Part model, mm, in its own coordinate system. A direction names the side the tool comes from. Round coordinates to 2 decimals unless told otherwise and drop trailing zeros. Order: outer loops, then holes, each group sorted by start corner. A loop starts at its lowest first (then second) coordinate and runs counter-clockwise, first axis right, second up. Notation, with made-up numbers: (49.5, 85) - (53.5, 85) arc R14 ccw to (53.5, 109) - close; hole circle Ø3 at (-6, -28.5). An arc over 180 degrees is marked (long way). Answer as a JSON object with one key per item and string values.
Autodesk Inventor part; units mm, degrees
ref_plane "Work Plane1" through (0, -10, 0) normal (0, 1, 0) x (-1, 0, 0)
ref_plane "YZ Plane" through (0, 0, 0) normal (1, 0, 0) x (0, 1, 0)
ref_plane "XY Plane" through (0, 0, 0) normal (0, 0, 1) x (1, 0, 0)
sketch "Sketch1" plane through (0, 0, 0) normal (1, 0, 0) x (0, 1, 0)
  circle A0 centre (0, 0) radius 7.5
  arc A1 (-3.1515, -19.7501) -> (-1.8071, 19.9182) centre (0, 0) ccw
  line L0 (-40, 20.115) -> (-40, -20.115)
  arc A2 (-40, 20.115) -> (-1.8071, 19.9182) centre (-19.8777, 219.1002) ccw
  arc A3 (-3.1515, -19.7501) -> (-40, -20.115) centre (-19.6039, -219.0723) ccw
  point P0 (-40, 0)
  dimension "d6" = 15
  dimension "d7" = 40
  dimension "d30" = 40.23
  dimension "d31" = 40
  dimension "d32" = 200
  dimension "d33" = 200
  dimension "d34" = 438.1724
  dimension "d35" = 219.0723
extrude "Extrusion1" add sketch "Sketch1" along normal mid plane 28
sketch "Sketch3" plane through (0, 0, 0) normal (0, 0, 1) x (1, 0, 0)
  line L0 (-14, 20) -> (14, 20) construction
  line L1 (-14, -3.1515) -> (14, -3.1515) construction
  line L2 (14, -40) -> (14, -3.1515) construction
  line L3 (14, -40) -> (-14, -40) construction
  line L4 (-14, -3.1515) -> (-14, -40) construction
  line L5 (-9, 20) -> (9, 20)
  line L6 (9, 20) -> (9, -10)
  line L7 (9, -10) -> (-9, -10)
  line L8 (-9, -10) -> (-9, 20)
  point P0 (0, 0)
  point P1 (0, 20)
  point P2 (0, 20)
  dimension "d19" = 18
  dimension "d21" = 10
extrude "Extrusion3" cut sketch "Sketch3" along normal through all both and the other way through all
ref_plane "Work Plane1" through (0, -10, 0) normal (0, 1, 0) x (-1, 0, 0)
sketch "Sketch5" plane through (0, -10, 0) normal (0, 1, 0) x (-1, 0, 0)
  circle A0 centre (0, 0) radius 2.75
  circle A1 centre (0, 0) radius 4.3
  dimension "d37" = 5.5
  dimension "d38" = 8.6
extrude "Extrusion6" cut sketch "Sketch5" against normal blind 3.2 contours A0 | A1
extrude "Extrusion7" cut sketch "Sketch5" against normal through all contours A0
properties part number "cabeza_obj1"
Item 1: Cut at A-A (z = 0). Write the cut outline in (x, y).
Taken from the geometry:
{"outline": "(-14, -40) - (-2.75, -40) - (-2.75, -13.2) - (-4.3, -13.2) - (-4.3, -10) - (-9, -10) - (-9, -7.5) - (-14, -7.5) - close; (-14, 7.5) - (-9, 7.5) - (-9, 20) - (-14, 20) - close; (2.75, -40) - (14, -40) - (14, -7.5) - (9, -7.5) - (9, -10) - (4.3, -10) - (4.3, -13.2) - (2.75, -13.2) - close; (9, 7.5) - (14, 7.5) - (14, 20) - (9, 20) - close"}
Item 2: Cut at C-C (y = 15). Write the cut outline in (x, z), plus the area to 3 significant figures.
Taken from the geometry:
{"outline": "(-14, -13.23) - (-9, -13.23) - (-9, 13.23) - (-14, 13.23) - close; (9, -13.23) - (14, -13.23) - (14, 13.23) - (9, 13.23) - close", "area": "265 mm2"}
Item 3: Tool access for faces 4 (the cylindrical face through (4.296, -11.578, 0.189)), 5 (the flat face through (-3, -40, 0)), 6 (the flat face through (9, 9, 0)): list every direction of +Z, -Z, +X, -X, +Y, -Y with a clear straight run to the whole face (end or side of a thin tool).
Taken from the geometry:
{"face 4": "+Y", "face 5": "+Z, -Z, +X, -X, -Y", "face 6": "+Z, -Z, +Y"}
Item 4: Cut at D-D (y = 0). Write the cut outline in (x, z), plus the area to 3 significant figures.
Taken from the geometry:
{"outline": "(-14, -20) - (-9, -20) - (-9, -7.5) - (-14, -7.5) - close; (-14, 7.5) - (-9, 7.5) - (-9, 20) - (-14, 20) - close; (9, -20) - (14, -20) - (14, -7.5) - (9, -7.5) - close; (9, 7.5) - (14, 7.5) - (14, 20) - (9, 20) - close", "area": "250 mm2"}
Item 5: Probe L1, parallel to X at y = 3, z = 9.5; L2, parallel to Y at x = -10.3, z = 0; L3, parallel to Y at x = -3, z = -6. List the from-to ranges inside material, lowest first. Write a range as from..to.
Taken from the geometry:
{"L1": "-14..-9, 9..14", "L2": "-40..-7.5, 7.5..20", "L3": "-40..-10"}
Item 6: Two-plate mould, pull along Y, no slides. Class faces 1 (the flat face through (0, -13.2, -3)), 2 (the cylindrical face through (-0.196, -21.842, -19.085)), 3 (the flat face through (-9, 8, 0)): pulls with the +Y half, pulls with the -Y half, needs draft (parallel to the pull), parting line crosses it, or undercut.
Taken from the geometry:
{"face 1": "pulls with the +Y half", "face 2": "undercut", "face 3": "needs draft"}
Item 7: Drop flat-ended pins along their axis: P1, Ø1, axis at x = 9.5, y = 2, coming from the -Z side; P2, Ø12, axis at x = 11, z = 13.5, coming from the +Y side; P3, Ø6, axis at x = -8, y = -23.5, coming from the -Z side. Give the stop position or say it passes through.
Taken from the geometry:
{"P1": "z = -19.94", "P2": "y = 18.54", "P3": "z = -19.19"}
